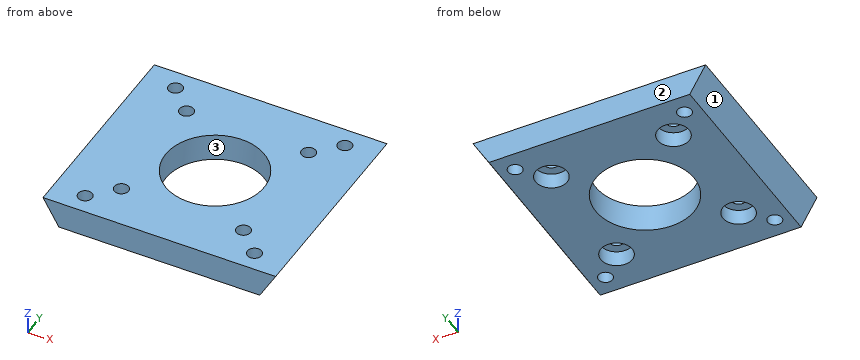
from build123d import *

# Parameters (mm, degrees)
SKETCH1_W               = 51
SKETCH1_H               = 53
BOSS_EXTRUDE1_DEPTH     = 7
CUT_EXTRUDE3_DEPTH      = 38.436613095
CUT_EXTRUDE3_DEPTH_BACK = 10
SKETCH2_R               = 12.5
SKETCH3_R               = 1.8
CUT_EXTRUDE4_DEPTH      = 10
SKETCH4_R               = 1.8
CUT_EXTRUDE5_DEPTH      = 11
BOSS_EXTRUDE2_DEPTH     = 53
SKETCH6_R               = 4
CUT_EXTRUDE6_DEPTH      = 4


with BuildPart() as part:
    # Sketch1 → Boss-Extrude1 (new body)
    with BuildSketch(Plane.XY):
        Rectangle(SKETCH1_W, SKETCH1_H)
    extrude(amount=BOSS_EXTRUDE1_DEPTH)

    # Sketch2 → Cut-Extrude3 (cut, two sides: drawn at the far end of the back side and taken through both)
    with BuildSketch(Plane.XY.offset(-CUT_EXTRUDE3_DEPTH_BACK)):
        with Locations(Location((0, 0, 0), (0, 0, 180))):
            Circle(SKETCH2_R)
    extrude(amount=CUT_EXTRUDE3_DEPTH + CUT_EXTRUDE3_DEPTH_BACK, mode=Mode.SUBTRACT)

    # Sketch3 → Cut-Extrude4 (cut)
    with BuildSketch(Plane.XY.offset(7)):
        with Locations((-15.5, 15.5)):
            Circle(SKETCH3_R)
        with Locations((15.5, 15.5)):
            Circle(SKETCH3_R)
        with Locations((15.5, -15.5)):
            Circle(SKETCH3_R)
        with Locations((-15.5, -15.5)):
            Circle(SKETCH3_R)
    extrude(amount=-CUT_EXTRUDE4_DEPTH, mode=Mode.SUBTRACT)

    # Sketch4 → Cut-Extrude5 (cut)
    with BuildSketch(Plane.XY.offset(7)):
        with Locations((-21.5, 21.5)):
            Circle(SKETCH4_R)
        with Locations((21.5, 21.5)):
            Circle(SKETCH4_R)
        with Locations((21.5, -21.5)):
            Circle(SKETCH4_R)
        with Locations((-21.5, -21.5)):
            Circle(SKETCH4_R)
    extrude(amount=-CUT_EXTRUDE5_DEPTH, mode=Mode.SUBTRACT)

    # Sketch5 → Boss-Extrude2 (add)
    with BuildSketch(Plane(origin=(0, 26.5, 0), x_dir=(1, 0, 0), z_dir=(0, 1, 0))):
        Polygon((-25.5, -7), (-29.541451884, -7), (-25.5, 0), align=None)
        Polygon((25.5, 0), (25.5, -7), (29.541451884, -7), align=None)
    extrude(amount=-BOSS_EXTRUDE2_DEPTH)

    # Sketch6 → Cut-Extrude6 (cut)
    with BuildSketch(Plane(origin=(0, 0, 0), x_dir=(-1, 0, 0), z_dir=(0, 0, -1))):
        with Locations((-15.5, 15.5)):
            Circle(SKETCH6_R)
        with Locations((15.5, 15.5)):
            Circle(SKETCH6_R)
        with Locations((15.5, -15.5)):
            Circle(SKETCH6_R)
        with Locations((-15.5, -15.5)):
            Circle(SKETCH6_R)
    extrude(amount=-CUT_EXTRUDE6_DEPTH, mode=Mode.SUBTRACT)


solid = part.part
Verification items for the finished model (mm, model axes). Face numbers are marked on the shaded views. Give positions to 0.01 mm unless a question says otherwise; leave off trailing zeros. Loops run counter-clockwise (first coordinate to the right, second up) from the corner with the lowest first, then second, coordinate; pieces in that order, holes last.
1) Sectioned sample at C-C, the plane y = 21.5. Enter the section's corners in (x, z), then the cut area to 3 significant figures.
2) Depth check by flat-ended pin: pin 1 Ø4 at (x, y) = (-15.5, 15.5) entering from -Z; pin 2 Ø4 at (y, z) = (-7.5, 4) entering from -X. Enter the tip coordinate at first touch or a pass-through.
3) Sectioned sample at B-B, the plane y = -7.5. Enter the section's corners in (x, z), then the cut area to 3 significant figures.
4) Sectioned sample at D-D, the plane z = 2. Count the separate pieces of the cut face and the enclosed holes in it, then the cut area to 3 significant figures.
5) Thickness scan on line 1 along Y through (x, z) = (-15.5, 4.6); line 2 along Y through (x, z) = (21.5, 5.5); line 3 along X through (y, z) = (2.5, 2.25). Record the ranges inside material, lowest first.
6) Sectioned sample at A-A, the plane x = 21.5. Enter the section's corners in (y, z).
7) Draft check along X on the marked faces 1, 2 and 3. Enter one of: pulls with the +X half, pulls with the -X half, needs draft (parallel to the pull), parting line crosses it, or undercut.
Answers:
1. outline: (-29.54, 7) - (-25.5, 0) - (-23.3, 0) - (-23.3, 7) - close; (-19.7, 0) - (19.7, 0) - (19.7, 7) - (-19.7, 7) - close; (23.3, 0) - (25.5, 0) - (29.54, 7) - (23.3, 7) - close
1. area: 335 mm2
2. pin 1: stops at z = 4
2. pin 2: stops at x = -28.96
3. outline: (-29.54, 7) - (-25.5, 0) - (-10, 0) - (-10, 7) - close; (10, 0) - (25.5, 0) - (29.54, 7) - (10, 7) - close
3. area: 245 mm2
4. separate pieces: 1
4. enclosed holes: 9
4. area: 2,090 mm2
5. line 1: y = -26.5 to -17.3, -13.7 to 13.7, 17.3 to 26.5
5. line 2: y = -26.5 to -23.3, -19.7 to 19.7, 23.3 to 26.5
5. line 3: x = -26.8 to -12.25, 12.25 to 26.8
6. outline: (-26.5, 0) - (-23.3, 0) - (-23.3, 7) - (-26.5, 7) - close; (-19.7, 0) - (19.7, 0) - (19.7, 7) - (-19.7, 7) - close; (23.3, 0) - (26.5, 0) - (26.5, 7) - (23.3, 7) - close
7. face 1: pulls with the -X half
7. face 2: needs draft
7. face 3: undercut
